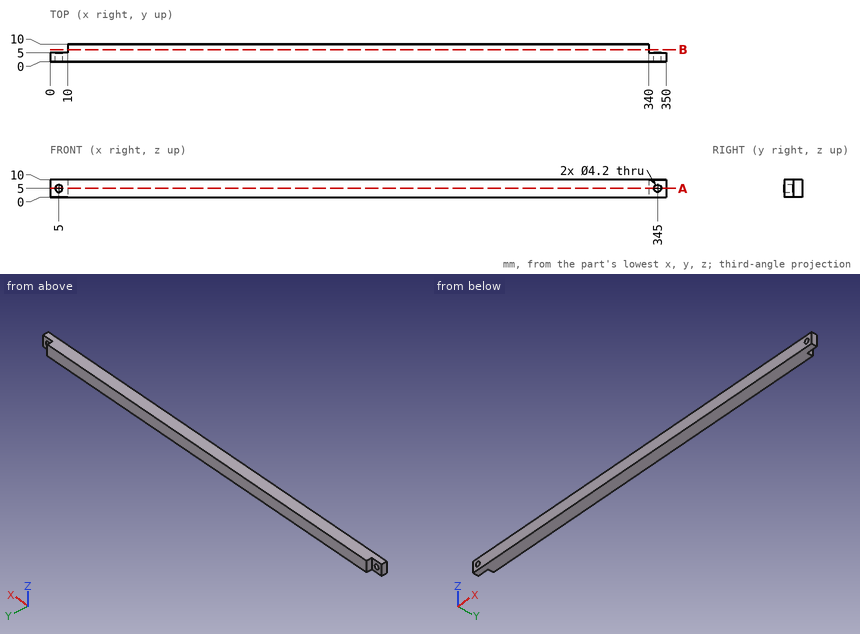
Source: three-view drawing plus pictorial views. Frame: mm from the lowest corner of the part. Coordinates: 2 decimals unless noted, no trailing zeros. Order: outer loops, then holes, each group sorted by start corner. A loop starts at its lowest first (then second) coordinate and runs counter-clockwise, first axis right, second up. Notation, with made-up numbers: M 43,16.5 L 100,16.5 A12 cw 100,35.5 Z; hole C 42,-20.5 d8. An arc over 180 degrees is marked long. Answer in a Markdown table with one row per item.
(1) Section query B-B, the plane y = 6.75. Output: boundary loops of the cut face in (x, z).
Numbers:
| item | result |
|---|---|
| outline | M 10,0 L 340,0 L 340,10 L 10,10 Z |
(2) Material intervals for line 1 (X direction, y = 4.75, z = 5); line 2 (Z direction, x = 345, y = 2.8); line 3 (X direction, y = 2, z = 6.5), sorted ascending. Write a range as [from, to].
Numbers:
| item | result |
|---|---|
| line 1 | x = [0, 2.9], [7.1, 342.9], [347.1, 350] |
| line 2 | z = [0, 2.9], [7.1, 10] |
| line 3 | x = [0, 3.53], [6.47, 343.53], [346.47, 350] |
(3) Section query A-A, the plane z = 5. Output: boundary loops of the cut face in (x, y).
Numbers:
| item | result |
|---|---|
| outline | M 0,0 L 2.9,0 L 2.9,5 L 0,5 Z; M 7.1,0 L 342.9,0 L 342.9,5 L 340,5 L 340,10 L 10,10 L 10,5 L 7.1,5 Z; M 347.1,0 L 350,0 L 350,5 L 347.1,5 Z |
(4) Contact query for flat-ended pins moving along their axis: pin 1 Ø4 at (y, z) = (9, 7.5) entering from +X; pin 2 Ø1.5 at (x, z) = (204, 7.5) entering from -Y; pin 3 Ø1 at (y, z) = (7.5, 2.5) entering from -X; pin 4 Ø2.5 at (x, z) = (345, 5) entering from -Y. Output: stop coordinate, or through.
Numbers:
| item | result |
|---|---|
| pin 1 | stops at x = 340 |
| pin 2 | stops at y = 0 |
| pin 3 | stops at x = 10 |
| pin 4 | passes through |
